The listing builds one solid part. Answer for the finished solid, in the listing's coordinates (mm). A direction names the side the tool comes from. Give positions to 0.01 mm unless a question says otherwise; leave off trailing zeros. Loops run counter-clockwise (first coordinate to the right, second up) from the corner with the lowest first, then second, coordinate; pieces in that order, holes last.
Item 1: Each of these flat-tipped pins is pushed along its axis until it touches: pin 1 Ø6.5 at (y, z) = (9.5, 3) entering from +X; pin 2 Ø6.5 at (y, z) = (8, 0) entering from -X; pin 3 Ø3.5 at (x, z) = (13, 1) entering from +Y. Where does it stop, or does it pass through?
Item 2: Section A-A, the plane x = -3 is taken. Give the vertices of the cut face in (y, z).
Item 3: Consider line 1 along Z through (x, y) = (-5.75, 8); line 2 along Z through (x, y) = (16, -15); line 3 along X through (y, z) = (0.6, -3). Determine where each line is inside the solid, lowest interval first.
Item 4: Section B-B, the plane y = 0.6 is taken. Give the vertices of the cut face in (x, z), and give its area (3 significant figures).
Item 5: A tool of negligible diameter and unlimited length cuts with its end or side. For faces 4 (the face through (-13.273, -16.358, -0.358)), 5 (the face through (-9, 0, 0)), 6 (the face through (0, -19.4, 0)), 7 (the face through (-0.5, 10.3, 0.1)), 8 (the face through (12, -13.4, 0)), from which of +Z, -Z, +X, -X, +Y, -Y can it reach the whole face along a straight path? Write none if from no direction.
Item 6: The mould has two halves that part along X. Classify faces 1 (the face through (9, 0, 0)), 2 (the face through (-0.213, -4.395, -0.098)), 3 (the face through (0, -10, 7)): pulls with the +X half, pulls with the -X half, needs draft (parallel to the pull), parting line crosses it, or undercut.
Item 7: Section C-C, the plane y = 8 is taken. Give the vertices of the cut face in (x, z), and give its area (3 significant figures).
Item 8: Section D-D, the plane z = 0 is taken. Give the number of separate pieces and of enclosed holes in the cut face, and give its area (4 significant figures).
from build123d import *

# Parameters (mm, degrees)
SKETCH_3_R          = 5
EXTRUDE_3_DEPTH     = 7
SKETCH_5_R          = 2.75
CUT_EXTRUDE_1_DEPTH = 10
SKETCH_6_W          = 1
SKETCH_6_H          = 13.139857665
CUT_EXTRUDE_2_DEPTH = 14
SKETCH_7_R          = 2
CUT_EXTRUDE_3_DEPTH = 37.405494091
HOLE_WIZARD_M4_1_D  = 3.3


with BuildPart() as part:
    # 草图3 → 凸台-拉伸3 (new, symmetric)
    with BuildSketch(Plane.XY):
        Polygon((-9, -13.4), (-21, -13.4), (-21, -19.4), (21, -19.4), (21, -13.4), (9, -13.4), (9, 13.4), (-9, 13.4), align=None)
        with Locations((0, 0.6)):
            Circle(SKETCH_3_R, mode=Mode.SUBTRACT)
    extrude(amount=EXTRUDE_3_DEPTH, both=True)

    # 草图5 → 切除-拉伸1 (cut)
    with BuildSketch(Plane(origin=(0, -13.4, 0), x_dir=(1, 0, 0), z_dir=(0, 1, 0))):
        with Locations(Location((-16, 0, 0), (0, 0, 270))):
            Circle(SKETCH_5_R)
        with Locations(Location((16, 0, 0), (0, 0, 180))):
            Circle(SKETCH_5_R)
    extrude(amount=-CUT_EXTRUDE_1_DEPTH, mode=Mode.SUBTRACT)

    # 草图6 → 切除-拉伸2 (cut)
    with BuildSketch(Plane.XY.offset(7)):
        with Locations((0, 10.029998353)):
            Rectangle(SKETCH_6_W, SKETCH_6_H)
    extrude(amount=-CUT_EXTRUDE_2_DEPTH, mode=Mode.SUBTRACT)

    # 草图7 → 切除-拉伸3 (cut, through all)
    with BuildSketch(Plane(origin=(9, 0, 0), x_dir=(0, 0, -1), z_dir=(1, 0, 0))):
        with Locations(Location((0, 8, 0), (0, 0, 90))):
            Circle(SKETCH_7_R)
    extrude(amount=-CUT_EXTRUDE_3_DEPTH, mode=Mode.SUBTRACT)

    # M4 螺纹孔1 (through all)
    with Locations(Plane.XY.offset(7)):
        with Locations((0, -14.9)):
            Hole(HOLE_WIZARD_M4_1_D / 2)


solid = part.part
Worked answers:
1. pin 1: stops at x = 9
1. pin 2: stops at x = -9
1. pin 3: stops at y = -13.4
2. outline: (-19.4, -7) - (-3.4, -7) - (-3.4, 7) - (-19.4, 7) - close; (4.6, -7) - (13.4, -7) - (13.4, 7) - (4.6, 7) - close; hole circle Ø4 at (8, 0)
3. line 1: z = -7 to -2, 2 to 7
3. line 2: z = -7 to -2.75, 2.75 to 7
3. line 3: x = -9 to -5, 5 to 9
4. outline: (-9, -7) - (-5, -7) - (-5, 7) - (-9, 7) - close; (5, -7) - (9, -7) - (9, 7) - (5, 7) - close
4. area: 112 mm2
5. face 4: +Y, -Y
5. face 5: +Z, -Z, -X, +Y
5. face 6: +Z, -Z, +X, -X, -Y
5. face 7: +Z, -Z, +Y
5. face 8: +Z, -Z, +X, +Y
6. face 1: pulls with the +X half
6. face 2: undercut
6. face 3: needs draft
7. outline: (-9, -7) - (-0.5, -7) - (-0.5, -2) - (-9, -2) - close; (-9, 2) - (-0.5, 2) - (-0.5, 7) - (-9, 7) - close; (0.5, -7) - (9, -7) - (9, -2) - (0.5, -2) - close; (0.5, 2) - (9, 2) - (9, 7) - (0.5, 7) - close
7. area: 170 mm2
8. separate pieces: 5
8. enclosed holes: 1
8. area: 505.5 mm2
